Check sheet for the modelled part. Datum: model origin and axes. Units: mm. Face numbers are marked on the shaded views. A direction names the side the tool comes from. Give positions to 0.01 mm unless a question says otherwise; leave off trailing zeros. Order: outer loops, then holes, each group sorted by start corner. A loop starts at its lowest first (then second) coordinate and runs counter-clockwise, first axis right, second up. Notation, with made-up numbers: (28.25, 84.5) -> (65.25, 84.5) arc R26 ccw to (65.25, 103.5) -> close; hole circle Ø8 at (-16, 18.5). An arc over 180 degrees is marked (long way). Answer in a Markdown table with one row per item. Add a question column.
(1) Cross-section at C-C (y = -0.75). Record the cut outline in (x, z).
(2) Release check for a two-part mould opening along X. For the marked faces 3, 4 and 5 record: released by +X, released by -X, zero draft, split by the parting line, or undercut.
(3) Cross-section at D-D (y = 2.5). Record the cut outline in (x, z), then the cut area to 3 significant figures.
(4) Cross-section at A-A (z = 0). Record the cut outline in (x, y).
(5) Set-up check for the marked faces 1 and 2: record each of +Z, -Z, +X, -X, +Y, -Y from which the full face is reachable in a straight line by a thin tool's end or side.
(6) Go/stop test with flat-tipped pins: pin 1 (2.5 mm diameter, centred on x = 0, z = 0, fed in from -Y); pin 2 (1.5 mm diameter, centred on x = -1.5, y = 6.5, fed in from -Z); pin 3 (4 mm diameter, centred on x = 5, y = 4.5, fed in from -Z); pin 4 (3.5 mm diameter, centred on x = 0, z = 0, fed in from +Y). Record where each tip stops, or that it passes through.
(7) Thickness scan on L1, parallel to X at y = 7.3, z = 0; L2, parallel to Y at x = -3.25, z = -4; L3, parallel to Z at x = 1, y = 7.5. Record the ranges inside material, lowest first. Write a range as [from, to].
(8) Cross-section at B-B (x = 0). Record the cut outline in (y, z), then the cut area to 3 significant figures.
```python
from build123d import *
from OCP.BRepFilletAPI import BRepFilletAPI_MakeChamfer

# Parameters (mm, degrees)
SKETCH1_R           = 8.5
BOSS_EXTRUDE1_DEPTH = 7.8
SKETCH2_R           = 8.5
SKETCH2_R_2         = 7.8
SKETCH2_R_3         = 1.5
CUT_EXTRUDE1_DEPTH  = 1.5
SKETCH3_R           = 0.5
BOSS_EXTRUDE2_DEPTH = 2
CHAMFER1_SIZE       = 0.5
CHAMFER1_SIZE2      = 0.1
FILLET1_R           = 1


with BuildPart() as part:
    # Sketch1 → Boss-Extrude1 (new body)
    with BuildSketch(Plane(origin=(0, 0, 0), x_dir=(1, 0, 0), z_dir=(0, 1, 0))):
        with Locations(Location((0, 0, 0), (0, 0, 270))):
            Circle(SKETCH1_R)
    extrude(amount=BOSS_EXTRUDE1_DEPTH)

    # Sketch2 → Cut-Extrude1 (cut)
    with BuildSketch(Plane(origin=(0, 7.8, 0), x_dir=(1, 0, 0), z_dir=(0, 1, 0))):
        with Locations(Location((0, 0, 0), (0, 0, 270))):
            Circle(SKETCH2_R)
        with Locations(Location((0, 0, 0), (0, 0, 270))):
            Circle(SKETCH2_R_2, mode=Mode.SUBTRACT)
        with Locations(Location((0, 0, 0), (0, 0, 270))):
            Circle(SKETCH2_R_3)
    extrude(amount=-CUT_EXTRUDE1_DEPTH, mode=Mode.SUBTRACT)

    # Sketch3 → Boss-Extrude2 (add)
    with BuildSketch(Plane.XZ):
        with Locations(Location((-5, 5, 0), (0, 0, 90))):
            Circle(SKETCH3_R)
        with Locations(Location((5, -5, 0), (0, 0, 90))):
            Circle(SKETCH3_R)
    extrude(amount=BOSS_EXTRUDE2_DEPTH)

    # Chamfer1: one chamfer whose edges measure the first distance from different faces: ONE call of the kernel's chamfer builder (chamfer() names one face for all edges)
    chamfer1_edges_1 = [part.edges().sort_by_distance(p)[0] for p in [
        (-5, -2, 4.5),
    ]]
    chamfer1_side_1 = [part.faces().sort_by_distance(p)[0] for p in [
        (-5, -1, 4.5),
    ]]
    chamfer1_edges_2 = [part.edges().sort_by_distance(p)[0] for p in [
        (5, -2, -5.5),
    ]]
    chamfer1_side_2 = [part.faces().sort_by_distance(p)[0] for p in [
        (5, -1, -5.5),
    ]]
    chamfer1 = BRepFilletAPI_MakeChamfer(part.part.solid().wrapped)
    for e in chamfer1_edges_1:
        chamfer1.Add(CHAMFER1_SIZE, CHAMFER1_SIZE2, e.wrapped, chamfer1_side_1[0].wrapped)  # the first distance lies on this face
    for e in chamfer1_edges_2:
        chamfer1.Add(CHAMFER1_SIZE, CHAMFER1_SIZE2, e.wrapped, chamfer1_side_2[0].wrapped)  # the first distance lies on this face
    add(Compound.cast(chamfer1.Shape()), mode=Mode.REPLACE)

    # Fillet1
    fillet1_edges = [part.edges().sort_by_distance(p)[0] for p in [
        (-5, -1.5, 4.5),
        (5, -1.5, -5.5),
    ]]
    fillet(fillet1_edges, radius=FILLET1_R)


solid = part.part
```
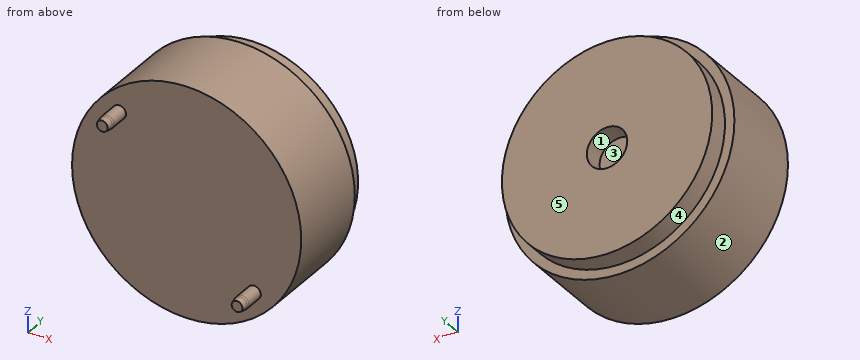
Answer below:
| question | item | result |
|---|---|---|
| 1 | outline | circle Ø1 at (-5, 5); circle Ø1 at (5, -5) |
| 2 | face 3 | undercut |
| 2 | face 4 | split by the parting line |
| 2 | face 5 | zero draft |
| 3 | outline | circle Ø17 at (0, 0) |
| 3 | area | 227 mm² |
| 4 | outline | (-8.5, 0) -> (8.5, 0) -> (8.5, 6.3) -> (7.8, 6.3) -> (7.8, 7.8) -> (1.5, 7.8) -> (1.5, 6.3) -> (-1.5, 6.3) -> (-1.5, 7.8) -> (-7.8, 7.8) -> (-7.8, 6.3) -> (-8.5, 6.3) -> close |
| 5 | face 1 | +Y |
| 5 | face 2 | +Y, -Y |
| 6 | pin 1 | stops at y = 0 |
| 6 | pin 2 | stops at z = -8.46 |
| 6 | pin 3 | stops at z = -7.95 |
| 6 | pin 4 | stops at y = 7.8 |
| 7 | L1 | x = [-7.8, -1.5], [1.5, 7.8] |
| 7 | L2 | y = [0, 7.8] |
| 7 | L3 | z = [-7.74, -1.12], [1.12, 7.74] |
| 8 | outline | (0, -8.5) -> (6.3, -8.5) -> (6.3, -7.8) -> (7.8, -7.8) -> (7.8, -1.5) -> (6.3, -1.5) -> (6.3, 1.5) -> (7.8, 1.5) -> (7.8, 7.8) -> (6.3, 7.8) -> (6.3, 8.5) -> (0, 8.5) -> close |
| 8 | area | 126 mm² |
